from build123d import *

# Parameters (mm, degrees)
F0_W     = 98.044
F0_H     = 98.044
F1_DEPTH = 15.24
F3_D     = 12.7
F2_W     = 4.572
F2_H     = 98.044
F2_W_2   = 44.45
F4_DEPTH = 0.7874


with BuildPart() as f1:
    # F0 (on Top) → F1 (new body)
    with BuildSketch(Plane.XY):
        Rectangle(F0_W, F0_H)
    extrude(amount=F1_DEPTH)

    # F3 (through all)
    with Locations(Plane.XY.offset(15.24)):
        with Locations((0, 0)):
            Hole(F3_D / 2)

    # F2 (on face) → F4 (cut)
    with BuildSketch(Plane.XY.offset(15.24)):
        with Locations((-46.736, 0)):
            Rectangle(F2_W, F2_H)
        with Locations((46.736, 0)):
            Rectangle(F2_W, F2_H)
        Rectangle(F2_W_2, F2_H)
    extrude(amount=-F4_DEPTH, mode=Mode.SUBTRACT)


solid = f1.part
Check sheet for the modelled part. Datum: model origin and axes. Units: mm. A direction names the side the tool comes from. Round coordinates to 2 decimals unless told otherwise and drop trailing zeros. Order: outer loops, then holes, each group sorted by start corner. A loop starts at its lowest first (then second) coordinate and runs counter-clockwise, first axis right, second up.
(1) Cross-section at A-A, the plane y = 0. Enter the section's corners in (x, z) (3 decimals), and give its area (3 significant figures).
(2) Cross-section at B-B, the plane x = 0. Enter the section's corners in (y, z), and give its area (3 significant figures).
(3) Access from +Z, -Z, +X, -X, +Y, -Y to the whole of each face (thin tool, end or side, straight path). Record for faces 1 (the flat face through (-12, 1, 0)), 2 (the flat face through (-47, 1, 14.453)), 3 (the flat face through (47, 1, 14.453)).
(4) Go/stop test with flat-tipped pins: P1, Ø11.5, axis at x = 0, y = 0, coming from the +Z side; P2, Ø1.4, axis at x = 47.5, y = 13, coming from the +Z side. Record where each tip stops, or that it passes through.
(5) Scan lines: probe 1 along Y at (x, z) = (0, 7.25); probe 2 along Z at (x, y) = (17.5, 8); probe 3 along Y at (x, z) = (4, 2.75). Record each from-to range of solid material in increasing order.
(6) Draft check along X on faces 4 (the flat face through (49.022, -1, 7)), 5 (the flat face through (10, 1, 14.453)), 6 (the flat face through (-1, -49.022, 8)), 7 (the cylindrical face through (1.38, -6.2, 7.13)). Enter one of: pulls with the +X half, pulls with the -X half, needs draft (parallel to the pull), parting line crosses it, or undercut.
(7) Cross-section at C-C, the plane y = 20. Enter the section's corners in (x, z) (3 decimals), and give its area (3 significant figures).
Check sheet entries:
1. outline: (-49.022, 0) - (-6.35, 0) - (-6.35, 14.453) - (-22.225, 14.453) - (-22.225, 15.24) - (-44.45, 15.24) - (-44.45, 14.453) - (-49.022, 14.453) - close; (6.35, 0) - (49.022, 0) - (49.022, 14.453) - (44.45, 14.453) - (44.45, 15.24) - (22.225, 15.24) - (22.225, 14.453) - (6.35, 14.453) - close
1. area: 1,270 mm2
2. outline: (-49.02, 0) - (-6.35, 0) - (-6.35, 14.45) - (-49.02, 14.45) - close; (6.35, 0) - (49.02, 0) - (49.02, 14.45) - (6.35, 14.45) - close
2. area: 1,230 mm2
3. face 1: -Z, +X, -X, +Y, -Y
3. face 2: +Z, -X, +Y, -Y
3. face 3: +Z, +X, +Y, -Y
4. P1: passes through
4. P2: stops at z = 14.45
5. probe 1: y = -49.02 to -6.35, 6.35 to 49.02
5. probe 2: z = 0 to 14.45
5. probe 3: y = -49.02 to -4.93, 4.93 to 49.02
6. face 4: pulls with the +X half
6. face 5: undercut
6. face 6: needs draft
6. face 7: undercut
7. outline: (-49.022, 0) - (49.022, 0) - (49.022, 14.453) - (44.45, 14.453) - (44.45, 15.24) - (22.225, 15.24) - (22.225, 14.453) - (-22.225, 14.453) - (-22.225, 15.24) - (-44.45, 15.24) - (-44.45, 14.453) - (-49.022, 14.453) - close
7. area: 1,450 mm2
